Input: part model. Units: mm. Frame: model coordinates. A direction names the side the tool comes from. Round coordinates to 2 decimals unless told otherwise and drop trailing zeros. Order: outer loops, then holes, each group sorted by start corner. A loop starts at its lowest first (then second) coordinate and runs counter-clockwise, first axis right, second up. Notation, with made-up numbers: (35.5, 45.25) -> (55.5, 45.25) arc R34 ccw to (55.5, 77.25) -> close; hole circle Ø1 at (44, 42.5). An arc over 180 degrees is marked (long way). Use a Markdown table: item, result.
from build123d import *

# Parameters (mm, degrees)
BOSS_EXTRUDE1_DEPTH        = 9
SKETCH11_R                 = 4.025
CUT_EXTRUDE4_DEPTH         = 7
CUT_EXTRUDE2_DEPTH         = 42.43669871
F_2_7_2_7_DIAMETER_HOLE1_D = 2.7


with BuildPart() as part:
    # Sketch1 → Boss-Extrude1 (new body)
    with BuildSketch(Plane.XY):
        with BuildLine():
            Line((-4.472135955, 4), (-20, 4))
            Line((-20, 4), (-20, -4))
            Line((-20, -4), (-4.472135955, -4))
            ThreePointArc((-4.472135955, -4), (0, -6), (4.472135955, -4))
            Line((4.472135955, -4), (20, -4))
            Line((20, -4), (20, 4))
            Line((20, 4), (4.472135955, 4))
            ThreePointArc((4.472135955, 4), (0, 6), (-4.472135955, 4))
        make_face()
    extrude(amount=BOSS_EXTRUDE1_DEPTH)

    # Sketch11 → Cut-Extrude4 (cut)
    with BuildSketch(Plane.XY.offset(9)):
        Circle(SKETCH11_R)
    extrude(amount=-CUT_EXTRUDE4_DEPTH, mode=Mode.SUBTRACT)

    # Sketch5 → Cut-Extrude2 (cut, through all)
    with BuildSketch(Plane.ZY.offset(20)):
        Polygon((0, 0), (2.183821406, -6), (0, -6), align=None)
    extrude(amount=-CUT_EXTRUDE2_DEPTH, mode=Mode.SUBTRACT)

    # Ø2.7 (2.7) Diameter Hole1 (through all)
    with Locations(Plane(origin=(0, 0, 0), x_dir=(-1, 0, 0), z_dir=(0, -0.34202014332566316, -0.9396926207859104))):
        with Locations((-16, -2.128355545), (16, -2.128355545)):
            Hole(F_2_7_2_7_DIAMETER_HOLE1_D / 2)


solid = part.part
1) Set-up query: faces 1 (the face through (12, 4, 4)), 2 (the face through (-12, -4, 5)), 3 (the face through (0, 0, 2)), 4 (the face through (12, -4, 5)), 5 (the face through (-12, 4, 4)). Return all of +Z, -Z, +X, -X, +Y, -Y with unobstructed straight access to the full face (end or side cutting, diameter ignored); none if empty.
Answer key:
| item | result |
|---|---|
| face 1 | +Z, -Z, +X, +Y |
| face 2 | +Z, -Z, -X, -Y |
| face 3 | +Z |
| face 4 | +Z, -Z, +X, -Y |
| face 5 | +Z, -Z, -X, +Y |
2) Draft query along Z for faces 6 (the face through (15.824, 0.887, 4.745)), 7 (the face through (0, 6, 4)), 8 (the face through (-0.28, -2.291, 0.834)). Return one class per face: released by +Z, released by -Z, zero draft, split by the parting line, or undercut.
Answer key:
| item | result |
|---|---|
| face 6 | undercut |
| face 7 | zero draft |
| face 8 | released by -Z |
3) Contact query for flat-ended pins moving along their axis: P1, Ø3, axis at x = 10.5, z = 4, coming from the +Y side; P2, Ø2.5, axis at x = 13, z = 3.5, coming from the -Y side; P3, Ø4, axis at x = -4, z = 6, coming from the +Y side. Output: stop coordinate, or through.
Answer key:
| item | result |
|---|---|
| P1 | stops at y = 4 |
| P2 | stops at y = -4 |
| P3 | stops at y = 5.66 |
4) Cut plane A-A on x = 0. Return loops of the section in (y, z) (3 decimals).
Answer key:
| item | result |
|---|---|
| outline | (-6, 2.184) -> (0, 0) -> (6, 0) -> (6, 9) -> (4.025, 9) -> (4.025, 2) -> (-4.025, 2) -> (-4.025, 9) -> (-6, 9) -> close |
5) Cut plane B-B on x = 11.5. Return loops of the section in (y, z), and give its area (3 significant figures).
Answer key:
| item | result |
|---|---|
| outline | (-4, 1.46) -> (0, 0) -> (4, 0) -> (4, 9) -> (-4, 9) -> close |
| area | 69.1 mm^2 |
6) Ray query, probe 1 along Y at (x, z) = (0, 6) (3 decimals); probe 2 along X at (y, z) = (-0.5, 1.5); probe 3 along Z at (x, y) = (1, 0.75). Return the intervals inside material, ascending.
Answer key:
| item | result |
|---|---|
| probe 1 | y = -6 to -4.025, 4.025 to 6 |
| probe 2 | x = -20 to -16.71, -15.29 to 15.29, 16.71 to 20 |
| probe 3 | z = 0 to 2 |
7) Cut plane C-C on z = 7. State how many separate pieces and enclosed holes the cut face has, and give its area (3 significant figures).
Answer key:
| item | result |
|---|---|
| separate pieces | 1 |
| enclosed holes | 3 |
| area | 282 mm^2 |
